Work out the finished part from the listing and answer in its coordinate system (mm). Face numbers are marked on the shaded views. A direction names the side the tool comes from. Give positions to 0.01 mm unless a question says otherwise; leave off trailing zeros. Loops run counter-clockwise (first coordinate to the right, second up) from the corner with the lowest first, then second, coordinate; pieces in that order, holes last. Notation, with made-up numbers: (28, 43) - (54, 43) arc R14 ccw to (54, 54) - close; hole circle Ø1 at (-33, 18.25). An arc over 180 degrees is marked (long way). Use one line per item in the form item = value. Start each with the question number.
from build123d import *

# Parameters (mm, degrees)
F0_W     = 133.35
F0_H     = 304.8
F0_R     = 2.182813
F1_DEPTH = 1.5875
F2_W     = 304.8
F2_H     = 304.8
F2_R     = 3.175
F3_DEPTH = 98.425
F4_W     = 298.45
F4_H     = 298.45
F5_DEPTH = 95.25
F6_W     = 304.8
F6_H     = 304.8
F6_W_2   = 279.4
F6_H_2   = 279.4
F7_DEPTH = 3.175
F8_R     = 2.38125
F9_DEPTH = 25.4


with BuildPart() as f1:
    # F0 (on Front) → F1 (new body)
    with BuildSketch(Plane.XZ):
        Rectangle(F0_W, F0_H)
        with Locations((-49.9745, -76.2)):
            Circle(F0_R, mode=Mode.SUBTRACT)
        with Locations((-42.1005, -76.2)):
            Circle(F0_R, mode=Mode.SUBTRACT)
        with Locations((42.1005, -76.2)):
            Circle(F0_R, mode=Mode.SUBTRACT)
        with Locations((49.9745, -76.2)):
            Circle(F0_R, mode=Mode.SUBTRACT)
        with Locations((-49.9745, 76.2)):
            Circle(F0_R, mode=Mode.SUBTRACT)
        with Locations((-42.1005, 76.2)):
            Circle(F0_R, mode=Mode.SUBTRACT)
        with Locations((42.1005, 76.2)):
            Circle(F0_R, mode=Mode.SUBTRACT)
        with Locations((49.9745, 76.2)):
            Circle(F0_R, mode=Mode.SUBTRACT)
    extrude(amount=F1_DEPTH)

    # F2 (on Front) → F3 (join)
    with BuildSketch(Plane.XZ):
        Rectangle(F2_W, F2_H)
        with Locations((-139.7, -114.3)):
            Circle(F2_R, mode=Mode.SUBTRACT)
        with Locations((-101.6, -101.6)):
            Circle(F2_R, mode=Mode.SUBTRACT)
        with Locations((139.7, -114.3)):
            Circle(F2_R, mode=Mode.SUBTRACT)
        with Locations((-139.7, 114.3)):
            Circle(F2_R, mode=Mode.SUBTRACT)
        with Locations((139.7, 114.3)):
            Circle(F2_R, mode=Mode.SUBTRACT)
    extrude(amount=-F3_DEPTH)

    # F4 (on face) → F5 (cut)
    with BuildSketch(Plane(origin=(0, 98.425, 0), x_dir=(-1, 0, 0), z_dir=(0, 1, 0))):
        Rectangle(F4_W, F4_H)
    extrude(amount=-F5_DEPTH, mode=Mode.SUBTRACT)

    # F6 (on face) → F7 (join)
    with BuildSketch(Plane(origin=(0, 98.425, 0), x_dir=(-1, 0, 0), z_dir=(0, 1, 0))):
        Rectangle(F6_W, F6_H)
        Rectangle(F6_W_2, F6_H_2, mode=Mode.SUBTRACT)
    extrude(amount=F7_DEPTH)

    # F8 (on face) → F9 (cut)
    with BuildSketch(Plane(origin=(0, 101.6, 0), x_dir=(-1, 0, 0), z_dir=(0, 1, 0))):
        with Locations((-146.05, 114.3)):
            Circle(F8_R)
        with Locations((146.05, 114.3)):
            Circle(F8_R)
        with Locations((146.05, -114.3)):
            Circle(F8_R)
        with Locations((-146.05, -114.3)):
            Circle(F8_R)
    extrude(amount=-F9_DEPTH, mode=Mode.SUBTRACT)


solid = f1.part
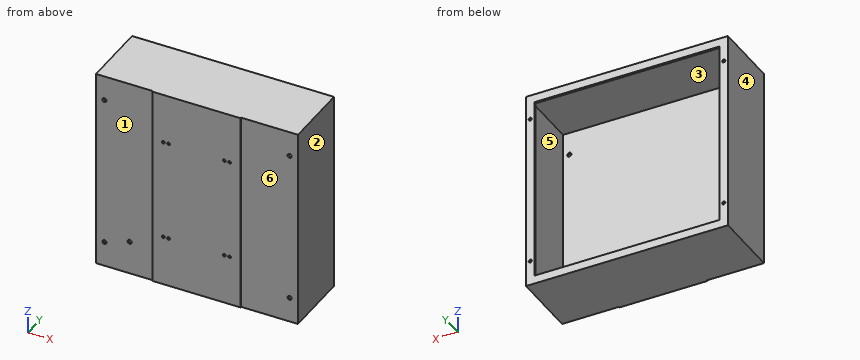
1) Determine the mould class of the marked faces 4, 5 and 6 for opening direction X: released by +X, released by -X, zero draft, split by the parting line, or undercut.
2) A cutting plane is placed at D-D (x = 29). Give the vertices of the cut face in (y, z) (1 decimal), plus the area to 3 significant figures.
3) Find the intervals of material crossed by probe 1 along Z at (x, y) = (139.7, 1.55) (3 decimals); probe 2 along Z at (x, y) = (139, 1); probe 3 along Z at (x, y) = (62, 37.5) (3 decimals), in increasing order.
4) A cutting plane is placed at A-A (y = 42). Give the vertices of the cut face in (x, z) (3 decimals).
5) A cutting plane is placed at C-C (z = 4.5). Give the vertices of the cut face in (x, y) (1 decimal), plus the area to 3 significant figures.
6) Flat-ended cylindrical pins translate along their axes: pin 1 Ø2 at (x, z) = (50.5, 76.5) entering from -Y; pin 2 Ø5 at (x, z) = (49.97, -76.2) entering from +Y (3 decimals); pin 3 Ø5 at (x, z) = (-101.6, -101.6) entering from -Y; pin 4 Ø0.5 at (y, z) = (-1, 10) entering from +X (3 decimals). Find the tip coordinate at first contact, or state that the pin passes through.
7) A tool of negligible diameter and unlimited length cuts with its end or side. For the marked faces 1, 2 and 3, from which of +Z, -Z, +X, -X, +Y, -Y can it reach the whole face along a straight path? Write none if from no direction.
8) A cutting plane is placed at B-B (x = 94). Give the vertices of the cut face in (y, z) (3 decimals).
Answer sheet:
q1.face_4 = released by -X
q1.face_5 = undercut
q1.face_6 = zero draft
q2.outline = (-1.6, -152.4) - (101.6, -152.4) - (101.6, -139.7) - (98.4, -139.7) - (98.4, -149.2) - (3.2, -149.2) - (3.2, 149.2) - (98.4, 149.2) - (98.4, 139.7) - (101.6, 139.7) - (101.6, 152.4) - (-1.6, 152.4) - close
q2.area = 2,140 mm²
q3.probe_1 = -152.4 to -117.475, -111.125 to 111.125, 117.475 to 152.4
q3.probe_2 = -152.4 to -117.4, -111.2 to 111.2, 117.4 to 152.4
q3.probe_3 = -152.4 to -149.225, 149.225 to 152.4
q4.outline = (-152.4, -152.4) - (152.4, -152.4) - (152.4, 152.4) - (-152.4, 152.4) - close; hole (-149.225, -149.225) - (149.225, -149.225) - (149.225, 149.225) - (-149.225, 149.225) - close
q5.outline = (-152.4, 0) - (-66.7, 0) - (-66.7, -1.6) - (66.7, -1.6) - (66.7, 0) - (152.4, 0) - (152.4, 101.6) - (139.7, 101.6) - (139.7, 98.4) - (149.2, 98.4) - (149.2, 3.2) - (-149.2, 3.2) - (-149.2, 98.4) - (-139.7, 98.4) - (-139.7, 101.6) - (-152.4, 101.6) - close
q5.area = 1,860 mm²
q6.pin_1 = 0
q6.pin_2 = 3.175
q6.pin_3 = through
q6.pin_4 = 66.675
q7.face_1 = +Z, -Z, -X, -Y
q7.face_2 = +Z, -Z, +X, +Y, -Y
q7.face_3 = none
q8.outline = (0, -152.4) - (101.6, -152.4) - (101.6, -139.7) - (98.425, -139.7) - (98.425, -149.225) - (3.175, -149.225) - (3.175, 149.225) - (98.425, 149.225) - (98.425, 139.7) - (101.6, 139.7) - (101.6, 152.4) - (0, 152.4) - close
